from build123d import *

# Parameters (mm, degrees)
PAD_DEPTH       = 5
SKETCH001_W     = 2
SKETCH001_H     = 12
POCKET_DEPTH    = 2
POCKET001_DEPTH = 4
SKETCH003_R     = 1.5
PAD001_DEPTH    = 4


with BuildPart() as part:
    # Sketch → Pad (new body)
    with BuildSketch(Plane.XY):
        Polygon((-28.5, 0), (28.5, 0), (28.5, 27.5), (30, 27.5), (30, 46), (-30, 46), (-30, 27.5), (-28.5, 27.5), align=None)
    extrude(amount=PAD_DEPTH)

    # Sketch001 (on Face9 of Pad) → Pocket (cut)
    with BuildSketch(Plane(origin=(0, 0, 0), x_dir=(1, 0, 0), z_dir=(0, 0, -1))):
        with Locations((-27.5, -6)):
            Rectangle(SKETCH001_W, SKETCH001_H)
        with Locations((27.5, -6)):
            Rectangle(SKETCH001_W, SKETCH001_H)
    extrude(amount=-POCKET_DEPTH, mode=Mode.SUBTRACT)

    # Sketch002 (on Face8 of Pocket) → Pocket001 (cut)
    with BuildSketch(Plane.XY.offset(5)):
        Polygon((-25.5, 0), (25.5, 0), (25.5, 13), (26.5, 13), (26.5, 46), (-26.5, 46), (-26.5, 13), (-25.5, 13), align=None)
    extrude(amount=-POCKET001_DEPTH, mode=Mode.SUBTRACT)

    # Sketch003 (on Face10 of Pocket001) → Pad001 (join)
    with BuildSketch(Plane.XY.offset(1)):
        with Locations((-10.5, 41)):
            Circle(SKETCH003_R)
        with Locations((10.5, 41)):
            Circle(SKETCH003_R)
    extrude(amount=PAD001_DEPTH)


solid = part.part
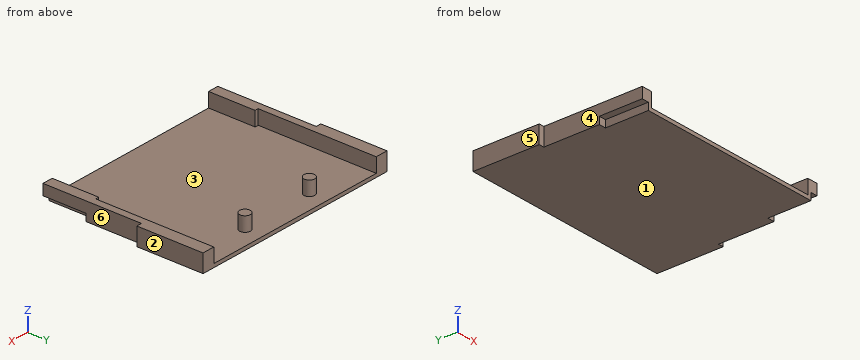
Input: part model. Units: mm. Frame: model coordinates. Face numbers are marked on the shaded views. A direction names the side the tool comes from. Coordinates: 2 decimals unless noted, no trailing zeros. Loops run counter-clockwise (first coordinate to the right, second up) from the corner with the lowest first, then second, coordinate; pieces in that order, holes last. Notation, with made-up numbers: (-26.75, 75) -> (5.25, 75) arc R7 ccw to (5.25, 83) -> close; hole circle Ø10 at (15.25, 11.25). An arc over 180 degrees is marked (long way). Write each question's results on one line, items separated by ' | '. Start each with the question number.
Q1. Section C-C, the plane x = -10.5. Return the cut outline in (y, z), plus the area to 3 significant figures.
Q2. Section B-B, the plane y = 14. Return the cut outline in (x, z), plus the area to 3 significant figures.
Q3. Ray query, line 1 (X direction, y = 31, z = 2.85); line 2 (X direction, y = 20.5, z = 3.6); line 3 (X direction, y = 40, z = 4.6). Return the intervals inside material, ascending. Write a range as from..to.
Q4. Section D-D, the plane y = 41. Return the cut outline in (x, z).
Q5. Pin query (flat end, axial travel): pin 1 (1.6 mm diameter, centred on x = -28, z = 1, fed in from -Y); pin 2 (2 mm diameter, centred on y = 7, z = 1.5, fed in from -X); pin 3 (4 mm diameter, centred on x = 21, y = 28.5, fed in from +Z). Return the tip coordinate at first contact, or that it passes through.
Q6. Reachability of the marked faces 4, 5 and 6 from +Z, -Z, +X, -X, +Y, -Y: full face, straight path, thin tool, end or side. Return the list, or none.
Q7. Pull-direction query (X, two-part tool) for the marked faces 1, 2 and 3; classes: released by +X, released by -X, zero draft, split by the parting line, or undercut.
Q8. Section A-A, the plane z = 2.8. Return the cut outline in (x, y).
Found:
1) outline: (0, 0) -> (46, 0) -> (46, 1) -> (42.5, 1) -> (42.5, 5) -> (39.5, 5) -> (39.5, 1) -> (0, 1) -> close | area: 58.0 mm2
2) outline: (-28.5, 0) -> (28.5, 0) -> (28.5, 5) -> (26.5, 5) -> (26.5, 1) -> (-26.5, 1) -> (-26.5, 5) -> (-28.5, 5) -> close | area: 73.0 mm2
3) line 1: -30..-26.5, 26.5..30 | line 2: -28.5..-26.5, 26.5..28.5 | line 3: -30..-26.5, -11.62..-9.38, 9.38..11.62, 26.5..30
4) outline: (-30, 0) -> (30, 0) -> (30, 5) -> (26.5, 5) -> (26.5, 1) -> (12, 1) -> (12, 5) -> (9, 5) -> (9, 1) -> (-9, 1) -> (-9, 5) -> (-12, 5) -> (-12, 1) -> (-26.5, 1) -> (-26.5, 5) -> (-30, 5) -> close
5) pin 1: y = 12 | pin 2: x = -28.5 | pin 3: z = 1
6) face 4: +Z, -Z, -X, -Y | face 5: +Z, -Z, -X, +Y, -Y | face 6: +Z, -Z, +X, -Y
7) face 1: zero draft | face 2: released by +X | face 3: undercut
8) outline: (-30, 27.5) -> (-28.5, 27.5) -> (-28.5, 0) -> (-25.5, 0) -> (-25.5, 13) -> (-26.5, 13) -> (-26.5, 46) -> (-30, 46) -> close; circle Ø3 at (-10.5, 41); circle Ø3 at (10.5, 41); (25.5, 0) -> (28.5, 0) -> (28.5, 27.5) -> (30, 27.5) -> (30, 46) -> (26.5, 46) -> (26.5, 13) -> (25.5, 13) -> close
